Autodesk Inventor part; units mm, degrees
ref_plane "Work Plane1" through (1.525, 0, 0) normal (0, 0, 1) x (1, 0, 0)
ref_plane "YZ Plane" through (0, 0, 0) normal (1, 0, 0) x (0, 1, 0)
ref_plane "XZ Plane" through (0, 0, 0) normal (0, 1, 0) x (-1, 0, 0)
sketch "Sketch1" plane through (0, 0, 0) normal (0, 0, 1) x (1, 0, 0)
  line L0 (0, 9.525) -> (0, 6.35)
  line L1 (38.1, 6.35) -> (69.85, 6.35)
  line L2 (69.85, 6.35) -> (69.85, 0)
  line L3 (69.85, 0) -> (-0.6351, 0)
  line L4 (-14.7321, 0) -> (83.947, 0)
  line L5 (-0.6351, 0) -> (-0.6351, 9.525)
  line L6 (-0.6351, 9.525) -> (0, 9.525)
  line L7 (38.1, 6.35) -> (25.8825, 6.35)
  line L8 (25.8825, 6.35) -> (0, 6.35)
  line L9 (0, -1.905) -> (0, 11.43)
  dimension "d0" = 69.85
  dimension "d1" = 31.75
  dimension "d2" = 12.7
  dimension "d9" = 0.6351
  dimension "d10" = 19.05
  dimension "d13" = 12.2175
  dimension "d14" = 12.7
revolve "Body" add sketch "Sketch1" angle 360 about axis through (69.85, 0, 0) along (-1, 0, 0)
sketch "Sketch2" plane through (-0.6351, 0, 0) normal (-1, 0, 0) x (0, 0, 1)
  line L0 (0, 10.9985) -> (9.525, 5.4993)
  line L1 (9.525, 5.4993) -> (9.525, -5.4993)
  line L2 (9.525, -5.4993) -> (0, -10.9985)
  line L3 (0, -10.9985) -> (-9.525, -5.4993)
  line L4 (-9.525, -5.4993) -> (-9.525, 5.4993)
  line L5 (-9.525, 5.4993) -> (0, 10.9985)
  point P0 (0, 0)
  point P1 (0, 0)
  dimension "d11" = 19.05
extrude "Head" add sketch "Sketch2" along normal blind 7.5692
sketch "Sketch4" plane through (0, 0, 0) normal (0, 0, 1) x (1, 0, 0)
  line L0 (-8.2043, 9.525) -> (-8.2043, 10.9985)
  line L1 (-8.2043, 10.9985) -> (-7.3536, 10.9985)
  line L2 (-7.3536, 10.9985) -> (-8.2043, 9.525)
  line L3 (-9.7181, 0) -> (0.8787, 0)
  line L4 (-0.6351, 10.9985) -> (-8.2043, 10.9985)
  line L5 (-8.2043, 5.4993) -> (-8.2043, 10.9985)
  dimension "d5" = 30
  dimension "d19" = 19.05
revolve "Chamfer1" cut sketch "Sketch4" angle 360 about axis through (-10, 0, 0) along (1, 0, 0)
thread "Thread"
chamfer "Chamfer2" distance 1.1985 distance2 1.1987 1 edges at (69.85, -6.35, 0) measured on face at (69.85, 1.2024, 1.742)
ref_plane "Work Plane1" through (1.525, 0, 0) normal (0, 0, 1) x (1, 0, 0)
equation "\"d0\" = NLG"
equation "\"d1\" = GEL"
equation "\"d2\" = GD"
equation "\"d10\" = SD2"
equation "\"d14\" = BDM"
equation "\"d11\" = SW"
equation "\"d3\" = KOH - SD"
equation "\"d5\" = ANG1"
equation "\"d19\" = SW0"
equation "\"d15\" = GEL"
equation "\"d6\" = -0.5 * SPD + 0.5 * GD"
equation "\"NLG\" = 69.85"
equation "\"GD\" = 12.7"
equation "\"BDM\" = 12.7"
equation "\"KOH\" = 8.2042"
equation "\"GEL\" = 31.75"
equation "\"SW\" = 19.05"
equation "\"SW0\" = SW"
equation "\"SPD\" = GD1"
equation "\"SD2\" = SW"
equation "\"SD\" = 0.635"
equation "\"ANG1\" = 30deg"
equation "\"GAL\" = 12.2174"
equation "\"GUL\" = 1.19863"
equation "\"RR\" = 0.381"
equation "\"WFT\" = SD"
equation "\"GD1\" = 10.303"
equation "\"THREADDIA\" = 12.7"
equation "\"SDH\" = SW"
equation "\"SDHG\" = 25.8826"
equation "\"TOA\" = 30deg"
equation "\"FAWI\" = 45deg"
equation "\"NND\" = 12.7"
equation "\"E0\" = 22.00275"
properties part number "AS 2465 - 1/2 x 2 3/4  UNC" material "Steel, Mild"
For this review, take the finished solid that the model builds, in its own axes (mm). A direction names the side the tool comes from. Coordinates: 2 decimals unless noted, no trailing zeros. Loops run counter-clockwise (first coordinate to the right, second up) from the corner with the lowest first, then second, coordinate; pieces in that order, holes last.
1. For line 1 (X direction, y = -7.5, z = 5.75); line 2 (Y direction, x = 33.5, z = -0.25); line 3 (Y direction, x = 19.5, z = -2), list the stretches that pass through material, from the lowest coordinate up.
2. Insertion check: P1, Ø6, axis at y = -8, z = 2, coming from the +X side; P2, Ø1.4, axis at y = -5, z = -7, coming from the +X side; P3, Ø1.5, axis at x = 31.5, y = -6, coming from the -Z side. Each pin has a flat end and moves straight along its axis. Give the tip position at first contact, or say it passes through.
3. Add section A-A, the plane x = -2. Give the boundary of the cut face in (y, z) (1 decimal).
4. For faces 1 (the flat face through (0, 6.2, 2)), 2 (the flat face through (-0.635, -5, -9)), 3 (the flat face through (-0.635, 5, -9)), list the 3-axis set-ups (+Z, -Z, +X, -X, +Y, -Y) from which the entire face can be reached by the end or side of a thin tool; tool diameter is ignored.
Result:
1. line 1: x = -8.2 to 0
1. line 2: y = -6.35 to 6.35
1. line 3: y = -6.03 to 6.03
2. P1: stops at x = 69.76
2. P2: stops at x = 0
2. P3: stops at z = -3.57
3. outline: (-11, 0) - (-5.5, -9.5) - (5.5, -9.5) - (11, 0) - (5.5, 9.5) - (-5.5, 9.5) - close
4. face 1: +X
4. face 2: -Z, +X, -Y
4. face 3: -Z, +X, +Y
